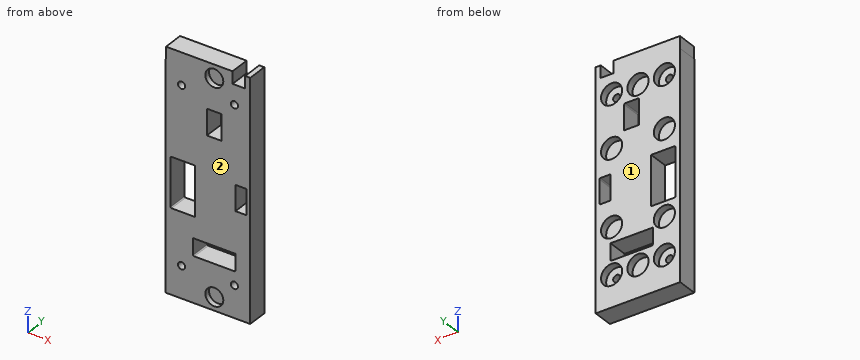
```python
from build123d import *

# Parameters (mm, degrees)
SKETCH1_W           = 80
SKETCH1_H           = 225
BOSS_EXTRUDE1_DEPTH = 19
CUT_EXTRUDE1_REACH  = 122.902
SKETCH4_R           = 10
CUT_EXTRUDE2_DEPTH  = 7
SKETCH5_R           = 8.5
CUT_EXTRUDE3_DEPTH  = 5
CUT_EXTRUDE4_REACH  = 122.902
SKETCH7_W           = 12
SKETCH7_H           = 11.5
SKETCH7_W_2         = 1
M8_TAPPED_HOLE1_D   = 6.8


with BuildPart() as part:
    # Sketch1 → Boss-Extrude1 (new body)
    with BuildSketch(Plane(origin=(0, 0, 0), x_dir=(1, 0, 0), z_dir=(0, 1, 0))):
        Rectangle(SKETCH1_W, SKETCH1_H)
    extrude(amount=-BOSS_EXTRUDE1_DEPTH)

    # Sketch2 → Cut-Extrude1 (cut, up to next)
    with BuildSketch(Plane(origin=(0, 0, 0), x_dir=(1, 0, 0), z_dir=(0, 1, 0)), mode=Mode.PRIVATE) as cut_extrude1_sk1:
        with BuildLine():
            Line((-34.5, -13.64), (-12.5, -13.64))
            Line((-12.5, -13.64), (-12.5, 33.36))
            Line((-12.5, 33.36), (-34.5, 33.36))
            ThreePointArc((-34.5, 33.36), (-35.207106781, 33.067106781), (-35.5, 32.36))
            Line((-35.5, 32.36), (-35.5, -12.64))
            ThreePointArc((-35.5, -12.64), (-35.207106781, -13.347106781), (-34.5, -13.64))
        make_face()
    cut_extrude1_tool1 = extrude(cut_extrude1_sk1.sketch, amount=-CUT_EXTRUDE1_REACH, mode=Mode.PRIVATE) & part.part
    # Sketch2 → Cut-Extrude1 (cut, up to next)
    with BuildSketch(Plane(origin=(0, 0, 0), x_dir=(1, 0, 0), z_dir=(0, 1, 0)), mode=Mode.PRIVATE) as cut_extrude1_sk2:
        with BuildLine():
            Line((0, -69.64), (12, -69.64))
            ThreePointArc((12, -69.64), (12.707106781, -69.347106781), (13, -68.64))
            Line((13, -68.64), (13, -45.14))
            Line((13, -45.14), (-1, -45.14))
            Line((-1, -45.14), (-1, -68.64))
            ThreePointArc((-1, -68.64), (-0.707106781, -69.347106781), (0, -69.64))
        make_face()
    cut_extrude1_tool2 = extrude(cut_extrude1_sk2.sketch, amount=-CUT_EXTRUDE1_REACH, mode=Mode.PRIVATE) & part.part
    # Sketch2 → Cut-Extrude1 (cut, up to next)
    with BuildSketch(Plane(origin=(0, 0, 0), x_dir=(1, 0, 0), z_dir=(0, 1, 0)), mode=Mode.PRIVATE) as cut_extrude1_sk3:
        with BuildLine():
            Line((35.5, 14.36), (26, 14.36))
            Line((26, 14.36), (26, -9.64))
            Line((26, -9.64), (35.5, -9.64))
            ThreePointArc((35.5, -9.64), (36.207106781, -9.347106781), (36.5, -8.64))
            Line((36.5, -8.64), (36.5, 13.36))
            ThreePointArc((36.5, 13.36), (36.207106781, 14.067106781), (35.5, 14.36))
        make_face()
    cut_extrude1_tool3 = extrude(cut_extrude1_sk3.sketch, amount=-CUT_EXTRUDE1_REACH, mode=Mode.PRIVATE) & part.part
    # Sketch2 → Cut-Extrude1 (cut, up to next)
    with BuildSketch(Plane(origin=(0, 0, 0), x_dir=(1, 0, 0), z_dir=(0, 1, 0)), mode=Mode.PRIVATE) as cut_extrude1_sk4:
        with BuildLine():
            Line((26, 53.36), (26, 68.64))
            ThreePointArc((26, 68.64), (25.707106781, 69.347106781), (25, 69.64))
            Line((25, 69.64), (-13, 69.64))
            ThreePointArc((-13, 69.64), (-13.707106781, 69.347106781), (-14, 68.64))
            Line((-14, 68.64), (-14, 53.36))
            Line((-14, 53.36), (26, 53.36))
        make_face()
    cut_extrude1_tool4 = extrude(cut_extrude1_sk4.sketch, amount=-CUT_EXTRUDE1_REACH, mode=Mode.PRIVATE) & part.part
    add(cut_extrude1_tool1.solids().sort_by_distance((-23.995521, 0, -9.86))[0], mode=Mode.SUBTRACT)
    add(cut_extrude1_tool2.solids().sort_by_distance((6, 0, 57.374932))[0], mode=Mode.SUBTRACT)
    add(cut_extrude1_tool3.solids().sort_by_distance((31.241424, 0, -2.36))[0], mode=Mode.SUBTRACT)
    add(cut_extrude1_tool4.solids().sort_by_distance((6, 0, -61.494779))[0], mode=Mode.SUBTRACT)

    # Sketch4 → Cut-Extrude2 (cut)
    with BuildSketch(Plane(origin=(0, 0, 0), x_dir=(1, 0, 0), z_dir=(0, 1, 0))):
        with Locations(Location((25, -82.5, 0), (0, 0, 270))):
            Circle(SKETCH4_R)
        with Locations(Location((0, -82.5, 0), (0, 0, 270))):
            Circle(SKETCH4_R)
        with Locations(Location((-25, -82.5, 0), (0, 0, 270))):
            Circle(SKETCH4_R)
        with Locations(Location((-25, -33, 0), (0, 0, 270))):
            Circle(SKETCH4_R)
        with Locations(Location((25, -33, 0), (0, 0, 270))):
            Circle(SKETCH4_R)
        with Locations(Location((25, 39, 0), (0, 0, 270))):
            Circle(SKETCH4_R)
        with Locations(Location((-25, 47, 0), (0, 0, 270))):
            Circle(SKETCH4_R)
        with Locations(Location((-25, 82.5, 0), (0, 0, 270))):
            Circle(SKETCH4_R)
        with Locations(Location((0, 82.5, 0), (0, 0, 270))):
            Circle(SKETCH4_R)
        with Locations(Location((25, 82.5, 0), (0, 0, 270))):
            Circle(SKETCH4_R)
    extrude(amount=-CUT_EXTRUDE2_DEPTH, mode=Mode.SUBTRACT)

    # Sketch5 → Cut-Extrude3 (cut)
    with BuildSketch(Plane.XZ.offset(19)):
        with Locations(Location((6, 100, 0), (0, 0, 270))):
            Circle(SKETCH5_R)
        with Locations(Location((6, -100, 0), (0, 0, 270))):
            Circle(SKETCH5_R)
    extrude(amount=-CUT_EXTRUDE3_DEPTH, mode=Mode.SUBTRACT)

    # Sketch7 → Cut-Extrude4 (cut, up to next)
    with BuildSketch(Plane(origin=(0, 0, 0), x_dir=(1, 0, 0), z_dir=(0, 1, 0)), mode=Mode.PRIVATE) as cut_extrude4_sk1:
        with Locations((29.25, -106.75)):
            Rectangle(SKETCH7_W, SKETCH7_H)
    cut_extrude4_tool1 = extrude(cut_extrude4_sk1.sketch, amount=-CUT_EXTRUDE4_REACH, mode=Mode.PRIVATE) & part.part
    # Sketch7 → Cut-Extrude4 (cut, up to next)
    with BuildSketch(Plane(origin=(0, 0, 0), x_dir=(1, 0, 0), z_dir=(0, 1, 0)), mode=Mode.PRIVATE) as cut_extrude4_sk2:
        with Locations((-40.25, -106.75)):
            Rectangle(SKETCH7_W_2, SKETCH7_H)
    cut_extrude4_tool2 = extrude(cut_extrude4_sk2.sketch, amount=-CUT_EXTRUDE4_REACH, mode=Mode.PRIVATE) & part.part
    add(cut_extrude4_tool1.solids().sort_by_distance((29.25, 0, 106.75))[0], mode=Mode.SUBTRACT)
    add(cut_extrude4_tool2.solids().sort_by_distance((-40.25, 0, 106.75))[0], mode=Mode.SUBTRACT)

    # M8 Tapped Hole1 (through all)
    with Locations(Plane(origin=(0, 0, 0), x_dir=(1, 0, 0), z_dir=(0, 1, 0))):
        with Locations((-25, 82.5), (25, 82.5), (25, -82.5), (-25, -82.5)):
            Hole(M8_TAPPED_HOLE1_D / 2)


solid = part.part
```
Design review of the part built by this model. Coordinates are the model's own, in mm. Face numbers are marked on the shaded views. Round coordinates to 2 decimals unless told otherwise and drop trailing zeros. Write each loop counter-clockwise with the first axis right and the second up, starting at its lowest first coordinate (ties: lowest second). Pieces come first, ordered by that corner, then holes. Notation, with made-up numbers: (68, 28) -> (84, 28) arc R23 ccw to (84, 66) -> close; hole circle Ø7 at (0, -36). An arc over 180 degrees is marked (long way). Write item = value, one per line. Start each with the question number.
1) Take a section at B-B, the plane z = -82.5. State the section outline as (x, y) points.
2) Mouldability with a two-part tool opening along Y and no side actions: class the marked faces 1 and 2 as +Y half, -Y half, draft (parallel to the pull), parting line (faces both ways), or undercut.
3) Take a section at A-A, the plane x = 33. State the section outline as (y, z) points, plus the area to 3 significant figures.
4) Clearance check with flat-ended pins moving along their axes: pin 1 (10 mm diameter, centred on x = 21.5, z = -41, fed in from +Y); pin 2 (7.5 mm diameter, centred on x = 30.5, y = -11, fed in from +Z). State where each tip first meets the part, or that it passes through.
5) Wall thickness on probe 1 along X at (y, z) = (-3.25, -82.5); probe 2 along Z at (x, y) = (1.5, -10.5); probe 3 along Z at (x, y) = (-30.5, -9.25): over which ranges is each line inside the solid? List them lowest first. Write a range as from..to.
6) Take a section at C-C, the plane x = 6. State the section outline as (y, z) points.
7) Take a section at D-D, the plane z = 33. State the section outline as (x, y) points.
Results list:
q1.outline = (-40, -19) -> (-28.4, -19) -> (-28.4, -7) -> (-35, -7) -> (-35, 0) -> (-40, 0) -> close; (-21.6, -19) -> (21.6, -19) -> (21.6, -7) -> (15, -7) -> (15, 0) -> (10, 0) -> (10, -7) -> (-10, -7) -> (-10, 0) -> (-15, 0) -> (-15, -7) -> (-21.6, -7) -> close; (28.4, -19) -> (40, -19) -> (40, 0) -> (35, 0) -> (35, -7) -> (28.4, -7) -> close
q2.face_1 = +Y half
q2.face_2 = -Y half
q3.outline = (-19, -112.5) -> (0, -112.5) -> (0, -88.5) -> (-7, -88.5) -> (-7, -76.5) -> (0, -76.5) -> (0, -45) -> (-7, -45) -> (-7, -33) -> (0, -33) -> (0, -14.36) -> (-19, -14.36) -> close; (-19, 9.64) -> (0, 9.64) -> (0, 27) -> (-7, 27) -> (-7, 39) -> (0, 39) -> (0, 76.5) -> (-7, 76.5) -> (-7, 88.5) -> (0, 88.5) -> (0, 101) -> (-19, 101) -> close
q3.area = 3,260 mm²
q4.pin_1 = -7
q4.pin_2 = 101
q5.probe_1 = -40..-35, -15..-10, 10..15, 35..40
q5.probe_2 = -112.5..-69.64, -53.36..45.14, 69.64..112.5
q5.probe_3 = -112.5..-33.36, 13.64..112.5
q6.outline = (-19, -112.5) -> (0, -112.5) -> (0, -90.5) -> (-7, -90.5) -> (-7, -74.5) -> (0, -74.5) -> (0, -69.64) -> (-19, -69.64) -> (-19, -91.5) -> (-14, -91.5) -> (-14, -108.5) -> (-19, -108.5) -> close; (-19, -53.36) -> (0, -53.36) -> (0, 45.14) -> (-19, 45.14) -> close; (-19, 69.64) -> (0, 69.64) -> (0, 74.5) -> (-7, 74.5) -> (-7, 90.5) -> (0, 90.5) -> (0, 112.5) -> (-19, 112.5) -> (-19, 108.5) -> (-14, 108.5) -> (-14, 91.5) -> (-19, 91.5) -> close
q7.outline = (-40, -19) -> (40, -19) -> (40, 0) -> (35, 0) -> (35, -7) -> (15, -7) -> (15, 0) -> (-15, 0) -> (-15, -7) -> (-35, -7) -> (-35, 0) -> (-40, 0) -> close
